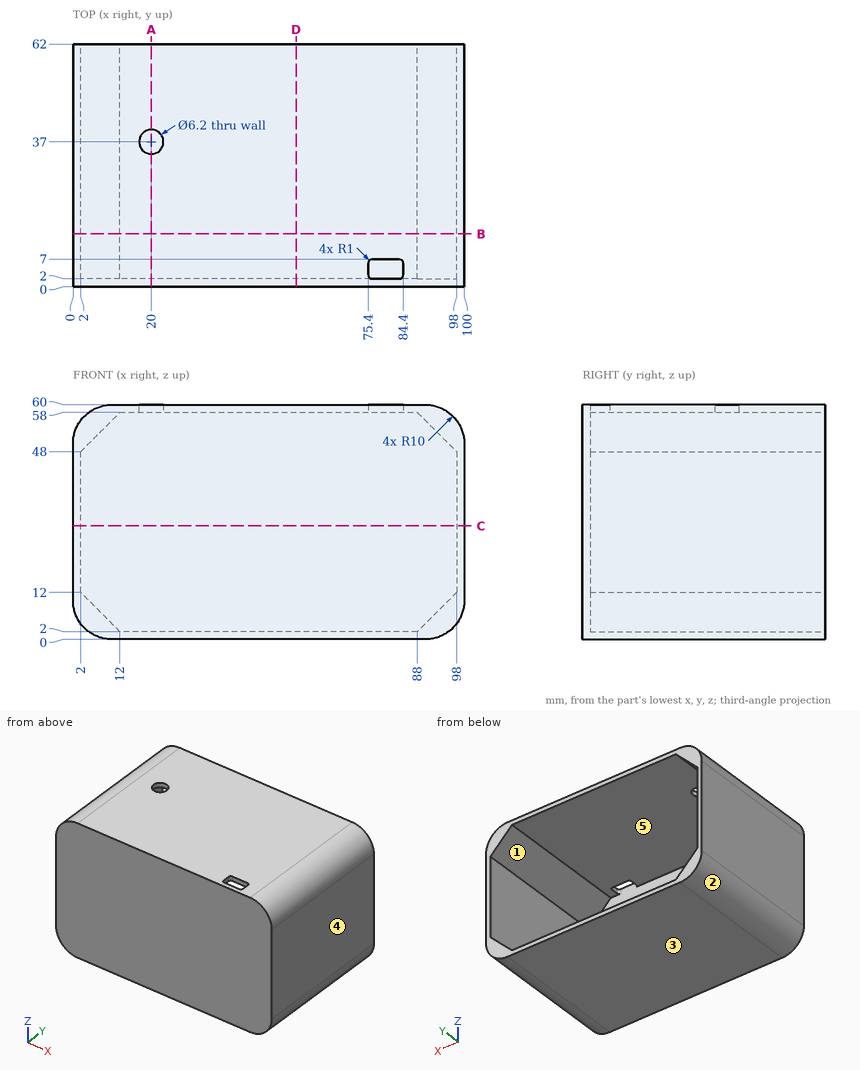
Source: three-view drawing plus pictorial views. Frame: mm from the lowest corner of the part. A direction names the side the tool comes from. Give positions to 0.01 mm unless a question says otherwise; leave off trailing zeros. Loops run counter-clockwise (first coordinate to the right, second up) from the corner with the lowest first, then second, coordinate; pieces in that order, holes last. Notation, with made-up numbers: M -32.5,2 L -28.5,2 A23 ccw -28.5,31 Z; hole C 76.5,-13 d3. An arc over 180 degrees is marked long. Put each result on its own line as item: value.
Q1. Pin query (flat end, axial travel): P1, Ø1, axis at y = 4.5, z = 58.5, coming from the +X side; P2, Ø2, axis at y = 5, z = 59, coming from the -X side. Return the tip coordinate at first contact, or that it passes through.
Response values:
P1: stops at x = 96
P2: stops at x = 4
Q2. Section C-C (z = 29). Return the cut outline in (x, y).
Response values:
outline: M 0,0 L 100,0 L 100,62 L 98,62 L 98,2 L 2,2 L 2,62 L 0,62 Z
Q3. Reachability of the marked faces 1 and 2 from +Z, -Z, +X, -X, +Y, -Y: full face, straight path, thin tool, end or side. Return the list, or none.
Response values:
face 1: +Y
face 2: -Z, -X, +Y, -Y
Q4. Section A-A (x = 20). Return the cut outline in (y, z).
Response values:
outline: M 0,0 L 62,0 L 62,2 L 2,2 L 2,58 L 33.9,58 L 33.9,60 L 0,60 Z; M 40.1,58 L 62,58 L 62,60 L 40.1,60 Z
Q5. Section B-B (y = 13.5). Return the cut outline in (x, z).
Response values:
outline: M 0,10 A10 ccw 10,0 L 90,0 A10 ccw 100,10 L 100,50 A10 ccw 90,60 L 10,60 A10 ccw 0,50 Z; hole M 2,12 L 12,2 L 88,2 L 98,12 L 98,48 L 88,58 L 12,58 L 2,48 Z
Q6. Line query: probe 1 along Z at (x, y) = (58.5, 43.5); probe 2 along X at (y, z) = (13.5, 12); probe 3 along Y at (x, z) = (20, 58.7). Output: solid intervals per line, ascending. Write a range as [from, to].
Response values:
probe 1: z = [0, 2], [58, 60]
probe 2: x = [0, 2], [98, 100]
probe 3: y = [0, 33.9], [40.1, 62]
Q7. Section D-D (x = 57). Return the cut outline in (y, z), and give its area (3 significant figures).
Response values:
outline: M 0,0 L 62,0 L 62,2 L 2,2 L 2,58 L 62,58 L 62,60 L 0,60 Z
area: 360 mm²
Q8. Mould query, pull axis X, two halves, no side actions, for the marked faces 3, 4 and 5. Classes: released by +X, released by -X, zero draft, split by the parting line, or undercut.
Response values:
face 3: zero draft
face 4: released by +X
face 5: undercut
